Can you work these out from the model? Positions are in its coordinate system, mm. Face numbers are marked on the shaded views. A direction names the side the tool comes from. Round coordinates to 2 decimals unless told otherwise and drop trailing zeros. Loops run counter-clockwise (first coordinate to the right, second up) from the corner with the lowest first, then second, coordinate; pieces in that order, holes last. Notation, with made-up numbers: M 6,10 L 65,10 A7 cw 65,22 Z; hole C 37.5,23 d6. An arc over 180 degrees is marked long. Use a Markdown table: item, result. Add a question column.
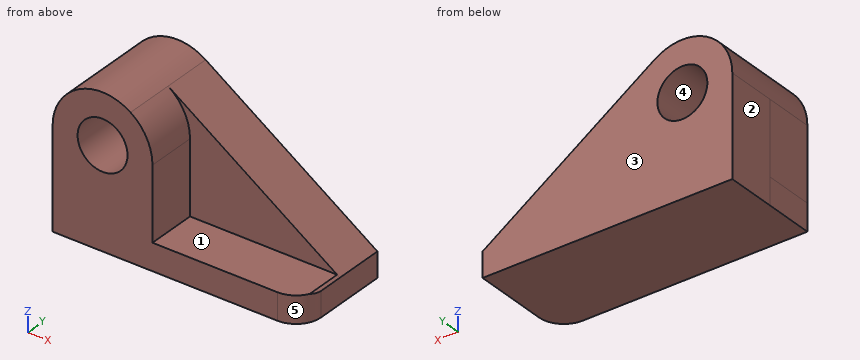
```python
from build123d import *

# Parameters (mm, degrees)
F0_R     = 12.7
F1_DEPTH = 25.4
F2_R     = 12.7
F3_DEPTH = 25.4
F4_R     = 12.7


# Not quite as in the source:
# - ends of sketch curves that miss each other by under 0.0002 mm in the source are joined


with BuildPart() as f1:
    # F0 (on Front) → F1 (new body)
    with BuildSketch(Plane.XZ):
        with BuildLine():
            Line((40.9585287035, -61.2564672112), (-46.4072367427, -2.1416516533))
            ThreePointArc((-46.4072367427, -2.1416516533), (-72.5399719473, -0.7377161417), (-86.0414712965, -23.1564672112))
            ThreePointArc((-86.0414712965, -23.1564672112), (-86.041478422, -23.1674516111), (-86.0414807971, -23.1784360131))
            Line((-86.0414807971, -23.1784360131), (-86.0414712965, -73.9564672112))
            Line((-86.0414712965, -73.9564672112), (40.9585287035, -73.9564672112))
            Line((40.9585287035, -73.9564672112), (40.9585287035, -61.2564672112))
        make_face()
        with Locations((-60.6414807971, -23.1784360131)):
            Circle(F0_R, mode=Mode.SUBTRACT)
    extrude(amount=F1_DEPTH)

    # F2 (on face) → F3 (join)
    with BuildSketch(Plane.XZ.offset(25.4)):
        with BuildLine():
            Line((-35.2414807971, -60.323882848), (-35.2414807971, -23.1784360131))
            ThreePointArc((-35.2414807971, -23.1784360131), (-38.2059086071, -11.2702413343), (-46.4072367427, -2.1416516533))
            ThreePointArc((-46.4072367427, -2.1416516533), (-72.5399719473, -0.7377161417), (-86.0414712965, -23.1564672112))
            ThreePointArc((-86.0414712965, -23.1564672112), (-86.041478422, -23.1674516111), (-86.0414807971, -23.1784360131))
            Line((-86.0414807971, -23.1784360131), (-86.0414712965, -60.323882848))
            Line((-86.0414712965, -60.323882848), (-86.0414712965, -73.9564672112))
            Line((-86.0414712965, -73.9564672112), (40.9585287035, -73.9564672112))
            Line((40.9585287035, -73.9564672112), (40.9585287035, -61.2564672112))
            Line((40.9585287035, -61.2564672112), (39.5802625959, -60.323882848))
            Line((39.5802625959, -60.323882848), (-35.2414807971, -60.323882848))
        make_face()
        with Locations((-60.6414807971, -23.1784360131)):
            Circle(F2_R, mode=Mode.SUBTRACT)
    extrude(amount=F3_DEPTH)

    # F4
    f4_edges = [f1.edges().sort_by_distance(p)[0] for p in [
        (40.958529, -50.8, -67.606467),
    ]]
    fillet(f4_edges, radius=F4_R)


solid = f1.part
```
(1) If I drill on probe 1 along Z at (x, y) = (0, -45); probe 2 along X at (y, z) = (-38, -46.5); probe 3 along Y at (x, z) = (-34, -57.5), over which ranges is the centre line in solid material (lowest first)? Write a range as [from, to].
(2) On a 3-axis mill with a long thin cutter (end or side, diameter ignored), from which of +Z, -Z, +X, -X, +Y, -Y can I reach the whole of each face in a straight line? I mean the marked faces 1 and 2. Say none if no direction works.
(3) Thinking about a two-plate mould opening in X: for the marked faces 3, 4 and 5, which applies, released by +X, released by -X, zero draft, split by the parting line, or undercut?
(4) Suppose I cut it at B-B on x = -59. List the corners of the cut face in (y, z) for me, and give its area (3 significant figures).
(5) Suppose I cut it at C-C on z = -17. List the corners of the cut face in (x, y) for me, and give its area (3 significant figures).
(6) I'm going to push flat-ended pins straight in: pin 1 (5 mm diameter, centred on x = 9, z = -45.5, fed in from -Y); pin 2 (2 mm diameter, centred on x = -34.5, y = -9, fed in from +Z); pin 3 (3 mm diameter, centred on x = 21.5, y = -36, fed in from +Z). Where does each tip first touch, or does it pass through?
(7) Suppose I cut it at D-D on x = -20. List the corners of the cut face in (y, z) for me.
Results below:
| question | item | result |
|---|---|---|
| 1 | probe 1 | z = [-73.96, -60.32] |
| 1 | probe 2 | x = [-86.04, -35.24] |
| 1 | probe 3 | y = [-25.4, 0] |
| 2 | face 1 | +Z, +X, -Y |
| 2 | face 2 | +Z, -Z, -X, +Y, -Y |
| 3 | face 3 | zero draft |
| 3 | face 4 | undercut |
| 3 | face 5 | released by +X |
| 4 | outline | M -50.8,-73.96 L 0,-73.96 L 0,-35.77 L -50.8,-35.77 Z; M -50.8,-10.58 L 0,-10.58 L 0,2.17 L -50.8,2.17 Z |
| 4 | area | 2,590 mm² |
| 5 | outline | M -85.28,-50.8 L -71.74,-50.8 L -71.74,0 L -85.28,0 Z; M -49.55,-50.8 L -36,-50.8 L -36,-25.4 L -24.45,-25.4 L -24.45,0 L -49.55,0 Z |
| 5 | area | 1,670 mm² |
| 6 | pin 1 | stops at y = -25.4 |
| 6 | pin 2 | stops at z = -9.52 |
| 6 | pin 3 | stops at z = -60.32 |
| 7 | outline | M -50.8,-73.96 L 0,-73.96 L 0,-20.01 L -25.4,-20.01 L -25.4,-60.32 L -50.8,-60.32 Z |
